from build123d import *

# Parameters (mm, degrees)
EXTRUDE1_DEPTH = 12.7


with BuildPart() as part:
    # Sketch1 → Extrude1 (new body)
    with BuildSketch(Plane.XY):
        with BuildLine():
            Line((95.25, 142.24), (63.5, 142.24))
            ThreePointArc((63.5, 142.24), (0, 205.74), (-63.5, 142.24))
            Line((-63.5, 142.24), (-95.25, 142.24))
            Line((-95.25, 142.24), (-95.25, 215.9))
            Line((-95.25, 215.9), (-53.975, 215.9))
            Line((-53.975, 215.9), (-53.975, 228.6))
            Line((-53.975, 228.6), (-34.925, 228.6))
            Line((-34.925, 228.6), (-34.925, 215.9))
            Line((-34.925, 215.9), (34.925, 215.9))
            Line((34.925, 215.9), (34.925, 228.6))
            Line((34.925, 228.6), (53.975, 228.6))
            Line((53.975, 228.6), (53.975, 215.9))
            Line((53.975, 215.9), (95.25, 215.9))
            Line((95.25, 215.9), (95.25, 142.24))
        make_face()
    extrude(amount=-EXTRUDE1_DEPTH)


solid = part.part
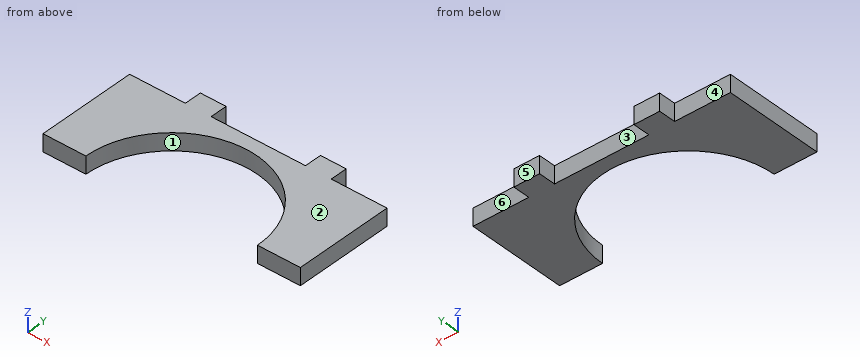
The listing builds one solid part. Answer for the finished solid, in the listing's coordinates (mm). Face numbers are marked on the shaded views. A direction names the side the tool comes from. Coordinates: 2 decimals unless noted, no trailing zeros. Loops run counter-clockwise (first coordinate to the right, second up) from the corner with the lowest first, then second, coordinate; pieces in that order, holes last. Notation, with made-up numbers: (48.25, 5) -> (91.25, 5) arc R34 ccw to (91.25, 37) -> close; hole circle Ø10 at (-12.75, -15.75). An arc over 180 degrees is marked (long way). Write item = value, one per line. Start each with the question number.
1) A cutting plane is placed at C-C (y = 190.5). Give the vertices of the cut face in (x, z).
2) The mould has two halves that part along X. Classify the marked faces 1 and 2: released by +X, released by -X, zero draft, split by the parting line, or undercut.
3) A cutting plane is placed at B-B (z = -6.5). Give the vertices of the cut face in (x, y) (3 decimals), then the cut area to 3 significant figures.
4) A tool of negligible diameter and unlimited length cuts with its end or side. For the marked faces 3, 4, 5 and 6, from which of +Z, -Z, +X, -X, +Y, -Y can it reach the whole face along a straight path? Write none if from no direction.
5) Straight lines are drawn through the part: line 1 (X direction, y = 222, z = -1.75) (3 decimals); line 2 (X direction, y = 171, z = -5.25); line 3 (Y direction, x = 52.5, z = -8). For each, find the intervals that lie inside material, in ascending order. Write a range as from..to.
6) A cutting plane is placed at A-A (y = 155). Give the vertices of the cut face in (x, z).
7) A cutting plane is placed at D-D (x = 0). Give the vertices of the cut face in (y, z), then the cut area to 3 significant figures.
8) Given pin 1 Ø3 at (x, z) = (-56.5, -3.5) entering from -Y; pin 2 Ø6 at (x, z) = (6, -3.5) entering from +Y; pin 3 Ø4 at (y, z) = (224, -4) entering from -X (3 decimals), each flat-ended and moving along its own axis, determine where each tip first touches the part or whether it passes through.
Responses:
q1.outline = (-95.25, -12.7) -> (-41.27, -12.7) -> (-41.27, 0) -> (-95.25, 0) -> close; (41.27, -12.7) -> (95.25, -12.7) -> (95.25, 0) -> (41.27, 0) -> close
q2.face_1 = undercut
q2.face_2 = zero draft
q3.outline = (-95.25, 142.24) -> (-63.5, 142.24) arc R63.5 cw to (63.5, 142.24) -> (95.25, 142.24) -> (95.25, 215.9) -> (53.975, 215.9) -> (53.975, 228.6) -> (34.925, 228.6) -> (34.925, 215.9) -> (-34.925, 215.9) -> (-34.925, 228.6) -> (-53.975, 228.6) -> (-53.975, 215.9) -> (-95.25, 215.9) -> close
q3.area = 8,180 mm²
q4.face_3 = +Z, -Z, +Y
q4.face_4 = +Z, -Z, -X, +Y
q4.face_5 = +Z, -Z, +X, -X, +Y
q4.face_6 = +Z, -Z, +X, +Y
q5.line_1 = -53.975..-34.925, 34.925..53.975
q5.line_2 = -95.25..-56.61, 56.61..95.25
q5.line_3 = 177.96..228.6
q6.outline = (-95.25, -12.7) -> (-62.2, -12.7) -> (-62.2, 0) -> (-95.25, 0) -> close; (62.2, -12.7) -> (95.25, -12.7) -> (95.25, 0) -> (62.2, 0) -> close
q7.outline = (205.74, -12.7) -> (215.9, -12.7) -> (215.9, 0) -> (205.74, 0) -> close
q7.area = 129 mm²
q8.pin_1 = 168.09
q8.pin_2 = 215.9
q8.pin_3 = -53.975
